The listing builds one solid part. Answer for the finished solid, in the listing's coordinates (mm). Face numbers are marked on the shaded views. Round coordinates to 2 decimals unless told otherwise and drop trailing zeros. Write each loop counter-clockwise with the first axis right and the second up, starting at its lowest first coordinate (ties: lowest second). Pieces come first, ordered by that corner, then holes. Notation, with made-up numbers: (79.5, 43.25) - (86.5, 43.25) arc R11 cw to (86.5, 57.25) - close; hole circle Ø7 at (36.5, 84.25). An arc over 180 degrees is marked (long way). Answer in a Markdown table with one row per item.
from build123d import *

# Parameters (mm, degrees)
ESBO_O1_R                = 7.5
RESSALTO_EXTRUS_O1_DEPTH = 12.5
ESBO_O7_R                = 2.5
CORTE_EXTRUS_O1_DEPTH    = 16
CORTE_EXTRUS_O2_DEPTH    = 28.156951228
FILETE2_R                = 0.3


with BuildPart() as part:
    # Esboço1 → Ressalto-extrusão1 (new, symmetric)
    with BuildSketch(Plane.XY):
        Circle(ESBO_O1_R)
    extrude(amount=RESSALTO_EXTRUS_O1_DEPTH, both=True)

    # Esboço7 → Corte-extrusão1 (cut)
    with BuildSketch(Plane(origin=(0, 0, 12.5), x_dir=(-1, 0, 0), z_dir=(0, 0, -1))):
        Circle(ESBO_O7_R)
    extrude(amount=CORTE_EXTRUS_O1_DEPTH, mode=Mode.SUBTRACT)

    # Esboço9 → Corte-extrusão2 (cut, through all)
    with BuildSketch(Plane.XY.offset(12.5)):
        Polygon((-0.75, 6), (-0.75, 7.5), (0.75, 7.5), (0.75, 6), (1.5, 6), (1.5, 4.5), (-1.5, 4.5), (-1.5, 6), align=None)
        Polygon((4.446152423, 4.299038106), (3.147114317, 3.549038106), (4.647114317, 0.950961894), (5.946152423, 1.700961894), (5.571152423, 2.350480947), (6.870190528, 3.100480947), (6.120190528, 4.399519053), (4.821152423, 3.649519053), align=None)
        Polygon((5.946152423, -1.700961894), (4.647114317, -0.950961894), (3.147114317, -3.549038106), (4.446152423, -4.299038106), (4.821152423, -3.649519053), (6.120190528, -4.399519053), (6.870190528, -3.100480947), (5.571152423, -2.350480947), align=None)
        Polygon((1.5, -6), (1.5, -4.5), (-1.5, -4.5), (-1.5, -6), (-0.75, -6), (-0.75, -7.5), (0.75, -7.5), (0.75, -6), align=None)
        Polygon((-4.446152423, -4.299038106), (-3.147114317, -3.549038106), (-4.647114317, -0.950961894), (-5.946152423, -1.700961894), (-5.571152423, -2.350480947), (-6.870190528, -3.100480947), (-6.120190528, -4.399519053), (-4.821152423, -3.649519053), align=None)
        Polygon((-5.946152423, 1.700961894), (-4.647114317, 0.950961894), (-3.147114317, 3.549038106), (-4.446152423, 4.299038106), (-4.821152423, 3.649519053), (-6.120190528, 4.399519053), (-6.870190528, 3.100480947), (-5.571152423, 2.350480947), align=None)
    extrude(amount=-CORTE_EXTRUS_O2_DEPTH, mode=Mode.SUBTRACT)

    # Filete2
    filete2_edges = [part.edges().sort_by_distance(p)[0] for p in [
        (-6.837632977, -3.081683836, 0),
        (-6.087632977, -4.380721942, 0),
        (-4.821152423, -3.649519053, 0),
        (-5.571152423, -2.350480947, 0),
        (-5.946152423, -1.700961894, 0),
        (-4.647114317, -0.950961894, 0),
        (-3.147114317, -3.549038106, 0),
        (-4.446152423, -4.299038106, 0),
        (-0.75, -7.462405778, 0),
        (0.75, -7.462405778, 0),
        (0.75, -6, 0),
        (-0.75, -6, 0),
        (-1.5, -6, 0),
        (-1.5, -4.5, 0),
        (1.5, -4.5, 0),
        (1.5, -6, 0),
        (6.087632977, -4.380721942, 0),
        (6.837632977, -3.081683836, 0),
        (5.571152423, -2.350480947, 0),
        (4.821152423, -3.649519053, 0),
        (4.446152423, -4.299038106, 0),
        (3.147114317, -3.549038106, 0),
        (4.647114317, -0.950961894, 0),
        (5.946152423, -1.700961894, 0),
        (6.837632977, 3.081683836, 0),
        (6.087632977, 4.380721942, 0),
        (4.821152423, 3.649519053, 0),
        (5.571152423, 2.350480947, 0),
        (5.946152423, 1.700961894, 0),
        (4.647114317, 0.950961894, 0),
        (3.147114317, 3.549038106, 0),
        (4.446152423, 4.299038106, 0),
        (0.75, 7.462405778, 0),
        (-0.75, 7.462405778, 0),
        (-0.75, 6, 0),
        (0.75, 6, 0),
        (1.5, 6, 0),
        (1.5, 4.5, 0),
        (-1.5, 4.5, 0),
        (-1.5, 6, 0),
        (-6.087632977, 4.380721942, 0),
        (-6.837632977, 3.081683836, 0),
        (-5.571152423, 2.350480947, 0),
        (-4.821152423, 3.649519053, 0),
        (-4.446152423, 4.299038106, 0),
        (-3.147114317, 3.549038106, 0),
        (-4.647114317, 0.950961894, 0),
        (-5.946152423, 1.700961894, 0),
    ]]
    fillet(filete2_edges, radius=FILETE2_R)


solid = part.part
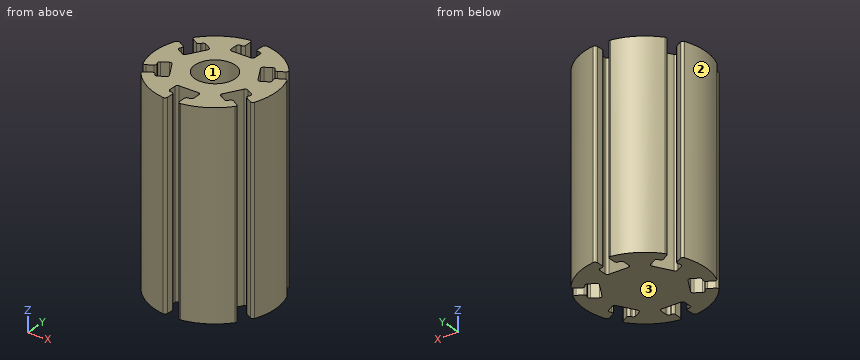
(1) Find the intervals of material crossed by line 1 (Y direction, x = 0, z = 1.5); line 2 (Y direction, x = 4.25, z = -10.25); line 3 (X direction, y = 2, z = 6.75), in increasing order.
Checked values:
| item | result |
|---|---|
| line 1 | y = -4.5 to -2.5, 2.5 to 4.5 |
| line 2 | y = -6.18 to -4.18, -1.64 to 1.64, 4.18 to 6.18 |
| line 3 | x = -7.23 to -5.77, -4.04 to -1.5, 1.5 to 4.04, 5.77 to 7.23 |
(2) Section A-A (y = 0) is taken. Give the vertices of the cut face in (x, z), and give its area (3 significant figures).
Checked values:
| item | result |
|---|---|
| outline | (-7.5, -12.5) - (7.5, -12.5) - (7.5, 12.5) - (2.5, 12.5) - (2.5, -3.5) - (-2.5, -3.5) - (-2.5, 12.5) - (-7.5, 12.5) - close |
| area | 295 mm2 |
(3) For a pull along X with two mould halves and no side action, classify the marked faces 1, 2 and 3 as pulls with the +X half, pulls with the -X half, needs draft (parallel to the pull), parting line crosses it, or undercut.
Checked values:
| item | result |
|---|---|
| face 1 | undercut |
| face 2 | pulls with the -X half |
| face 3 | needs draft |
(4) Flat-ended cylindrical pins translate along their axes: pin 1 (0.7 mm diameter, centred on y = 5.5, z = -5, fed in from -X); pin 2 (0.9 mm diameter, centred on y = 6.5, z = 5.5, fed in from -X); pin 3 (0.9 mm diameter, centred on y = -7, z = -2, fed in from +X); pin 4 (2.5 mm diameter, centred on x = 1, y = -1, fed in from +Z). Find the tip coordinate at first contact, or state that the pin passes through.
Checked values:
| item | result |
|---|---|
| pin 1 | stops at x = -5.45 |
| pin 2 | stops at x = -4.43 |
| pin 3 | stops at x = 3.65 |
| pin 4 | stops at z = 12.5 |
(5) Section B-B (x = 0) is taken. Give the vertices of the cut face in (y, z).
Checked values:
| item | result |
|---|---|
| outline | (-4.5, -12.5) - (4.5, -12.5) - (4.5, 12.5) - (2.5, 12.5) - (2.5, -3.5) - (-2.5, -3.5) - (-2.5, 12.5) - (-4.5, 12.5) - close |
